```python
from build123d import *

# Parameters (mm, degrees)
F0_W      = 81.1027027667
F0_H      = 39.3372392282
F1_DEPTH  = 8.636
F3_DEPTH  = 25.4
F4_W      = 79.281533137
F4_H      = 5.9491507709
F5_DEPTH  = 25.4
F6_W      = 6.7990301177
F6_H      = 35.5734908953
F7_DEPTH  = 25.4
F9_DEPTH  = 25.4
F10_R     = 4.4646843998
F10_R_2   = 4.4902635422
F11_DEPTH = 25.4
F13_DEPTH = 25.4


with BuildPart() as f1:
    # F0 (on Front) → F1 (new body)
    with BuildSketch(Plane.XZ):
        with Locations((-8.7416078895, 6.434794981)):
            Rectangle(F0_W, F0_H)
    extrude(amount=F1_DEPTH)

    # F2 (on face) → F3 (cut)
    with BuildSketch(Plane.XZ.offset(8.636)):
        Polygon((-49.2929592729, -13.2338246331), (-10.5112984066, -13.2338246331), (-49.2929592729, 14.1543564849), align=None)
    extrude(amount=-F3_DEPTH, mode=Mode.SUBTRACT)

    # F4 (on face) → F5 (join)
    with BuildSketch(Plane.XZ.offset(8.636)):
        with Locations((-9.6521927044, 23.1288392097)):
            Rectangle(F4_W, F4_H)
    extrude(amount=F5_DEPTH)

    # F6 (on face) → F7 (join)
    with BuildSketch(Plane.XZ.offset(8.636)):
        with Locations((3.3995150588, 2.3675183766)):
            Rectangle(F6_W, F6_H)
    extrude(amount=F7_DEPTH)

    # F8 (on face) → F9 (cut)
    with BuildSketch(Plane.YZ.offset(6.7990301177)):
        Polygon((-34.036, -15.4192270711), (-9.674085426, -15.4192270711), (-34.036, 9.5568542875), align=None)
    extrude(amount=-F9_DEPTH, mode=Mode.SUBTRACT)

    # F10 (on face) → F11 (cut)
    with BuildSketch(Plane.XZ.offset(8.636)):
        with Locations((12.8695918247, 0)):
            Circle(F10_R)
        with Locations((25.7391780615, 0)):
            Circle(F10_R_2)
    extrude(amount=-F11_DEPTH, mode=Mode.SUBTRACT)

    # F12 (on face) → F13 (cut)
    with BuildSketch(Plane.XY.offset(26.1034145951)):
        Polygon((29.9885738641, -34.036), (29.9885738641, -12.5484813482), (7.9453402096, -34.036), align=None)
    extrude(amount=-F13_DEPTH, mode=Mode.SUBTRACT)


solid = f1.part
```
Model file for the job. Use its own axes, mm. A direction names the side the tool comes from. Coordinates: 2 decimals unless noted, no trailing zeros. Order: outer loops, then holes, each group sorted by start corner. A loop starts at its lowest first (then second) coordinate and runs counter-clockwise, first axis right, second up. Notation, with made-up numbers: (-36, 37.5) -> (14, 37.5) arc R27 ccw to (14, 62.5) -> close; hole circle Ø10 at (83, 57.25). An arc over 180 degrees is marked (long way). Answer as a JSON object with one key per item and string values. Group by question number.
1) Cut at D-D, the plane y = -19. Write the cut outline in (x, z), then the cut area to 3 significant figures.
2) Flat gauge pins, fed straight in: pin 1 (7.5 mm diameter, centred on x = -32, y = -18.5, fed in from -Z); pin 2 (0.7 mm diameter, centred on x = 4.5, z = -14.5, fed in from +Y); pin 3 (2 mm diameter, centred on y = -13, z = -8, fed in from +X). Where does each tip first touch, or does it go through?
3) Cut at A-A, the plane y = -7. Write the cut outline in (x, z), then the cut area to 3 significant figures.
4) Cut at C-C, the plane z = 0. Write the cut outline in (x, y).
5) Drill centre lines: L1, parallel to Z at x = -0.5, y = -2.5; L2, parallel to Z at x = -19.5, y = -21; L3, parallel to X at y = -18, z = 0. Where is each one in solid material? Low to high.
6) Cut at B-B, the plane x = 24.5. Write the cut outline in (y, z), then the cut area to 3 significant figures.
7) Which spindle directions (+Z, -Z, +X, -X, +Y, -Y) get a long thin tool onto all of the face, cutting with end or side? Do faces 1 (the face through (16, -18, 20.154)), 2 (the face through (29.989, -11, 23)), 3 (the face through (3, -8.636, -14)), 4 (the face through (-20, -8.636, 7)), 5 (the face through (3.45, -21.68, -3.11)). Say none if no direction does.
8) Pull direction X, two halves, no side cores. Call faces 6 (the face through (0, -18, 6)), 7 (the face through (17, -4.4, -1.7)), 8 (the face through (0, 0, 11)), 9 (the face through (19.121, -23.142, 23.17)): +X half, -X half, draft (parallel to the pull), parting line (faces both ways), or undercut.
Check values:
{
 "1": {"outline": "(-49.29, 20.15) -> (0, 20.15) -> (0, -5.86) -> (6.8, -5.86) -> (6.8, 20.15) -> (23.37, 20.15) -> (23.37, 26.1) -> (-49.29, 26.1) -> close", "area": "609 mm²"},
 "2": {"pin 1": "stops at z = 20.15", "pin 2": "stops at y = -8.64", "pin 3": "stops at x = 6.8"},
 "3": {"outline": "(-49.29, 14.15) -> (-10.51, -13.23) -> (31.81, -13.23) -> (31.81, 26.1) -> (-49.29, 26.1) -> close; hole circle Ø8.93 at (12.87, 0); hole circle Ø8.98 at (25.74, 0)", "area": "2,530 mm²"},
 "4": {"outline": "(-29.25, -8.64) -> (0, -8.64) -> (0, -24.71) -> (6.8, -24.71) -> (6.8, -8.64) -> (8.4, -8.64) -> (8.4, 0) -> (-29.25, 0) -> close; (17.33, -8.64) -> (21.25, -8.64) -> (21.25, 0) -> (17.33, 0) -> close; (30.23, -8.64) -> (31.81, -8.64) -> (31.81, 0) -> (30.23, 0) -> close"},
 "5": {"L1": "z = -13.23 to 26.1", "L2": "z = 20.15 to 26.1", "L3": "x = 0 to 6.8"},
 "6": {"outline": "(-17.9, 20.15) -> (-8.64, 20.15) -> (-8.64, 4.32) -> (0, 4.32) -> (0, 26.1) -> (-17.9, 26.1) -> close; (-8.64, -13.23) -> (0, -13.23) -> (0, -4.32) -> (-8.64, -4.32) -> close", "area": "320 mm²"},
 "7": {"face 1": "-Z, +X, -Y", "face 2": "+Z, -Z, +X, -Y", "face 3": "-Z, +X, -X, +Y", "face 4": "-Z, -X, -Y", "face 5": "-Z, +X, -X, -Y"},
 "8": {"face 6": "-X half", "face 7": "undercut", "face 8": "draft", "face 9": "+X half"}
}
